Read the model definition and answer for the solid it produces. Units are mm, in the model's axes. A direction names the side the tool comes from. Give positions to 0.01 mm unless a question says otherwise; leave off trailing zeros. Write each loop counter-clockwise with the first axis right and the second up, starting at its lowest first coordinate (ties: lowest second). Pieces come first, ordered by that corner, then holes. Notation, with made-up numbers: (20.5, 34) - (65.5, 34) arc R6 cw to (65.5, 43) - close; hole circle Ø8 at (71, 61). An arc over 180 degrees is marked (long way). Use CSV: the item, a comma, the result in double quotes. Start each with the question number.
from build123d import *

# Parameters (mm, degrees)
SKETCH_1_R               = 4
EXTRUDE_1_DEPTH          = 2
SKETCH_6_R               = 6
EXTRUDE_3_DEPTH          = 1
SKETCH_2_R               = 0.5
CUT_EXTRUDE_1_DEPTH      = 2
PATTERN_CIRCULAR_1_COUNT = 3
CHAMFER_1_SIZE           = 0.5
EXTRUDE_START            = -2
EXTRUDE_4_DEPTH          = 2
HOLE_WIZARD_M3_1_D       = 3.4
SKETCH_11_R              = 3.5
CUT_EXTRUDE_3_DEPTH      = 1
CUT_EXTRUDE_4_DEPTH      = 29.574464124
FILLET_1_R               = 1
FILLET_2_R               = 1


with BuildPart() as part:
    # ｽｹｯﾁ1 → ﾎﾞｽ - 押し出し1 (new body)
    with BuildSketch(Plane.XY):
        with BuildLine():
            ThreePointArc((-4.5, -6), (7.5, 0), (-4.5, 6))
            ThreePointArc((-4.5, 6), (-7.5, 5), (-10.5, 6))
            ThreePointArc((-10.5, 6), (-22.5, 0), (-10.5, -6))
            ThreePointArc((-10.5, -6), (-7.5, -5), (-4.5, -6))
        make_face()
        Circle(SKETCH_1_R, mode=Mode.SUBTRACT)
    extrude(amount=EXTRUDE_1_DEPTH)

    # ｽｹｯﾁ6 → ﾎﾞｽ - 押し出し3 (add)
    with BuildSketch(Plane.XY.offset(2)):
        with Locations((-15, 0)):
            Circle(SKETCH_6_R)
    extrude(amount=EXTRUDE_3_DEPTH)

    # ｽｹｯﾁ2 → ｶｯﾄ - 押し出し1 (cut)
    with BuildSketch(Plane.XY.offset(3)):
        with Locations((-11.5, 0)):
            Circle(SKETCH_2_R)
    extrude(amount=-CUT_EXTRUDE_1_DEPTH, mode=Mode.SUBTRACT)

    # ｽｹｯﾁ4 → M3x0.5 ねじ穴1 (revolve, cut)
    with BuildSketch(Plane(origin=(-11.5, 0, 3), x_dir=(0, -1, 0), z_dir=(1, 0, 0))):
        Polygon((0, 0), (0, 3), (1.525, 3), (1.25, 2.725), (1.25, 0.025), (1.275, 0), align=None)
    m3x0_5_1 = revolve(axis=Axis((-11.5, 0, 9.35), (0, 0, -1)), mode=Mode.SUBTRACT)

    # 円形ﾊﾟﾀｰﾝ1: M3x0.5 ねじ穴1 ×3 about axis
    pattern_circular_1_axis = Axis((-15, 0, 0), (0, 0, 1))
    for i in range(1, PATTERN_CIRCULAR_1_COUNT):
        add(m3x0_5_1.rotate(pattern_circular_1_axis, i * 360 / PATTERN_CIRCULAR_1_COUNT), mode=Mode.SUBTRACT)

    # 面取り1
    chamfer_1_edges = [part.edges().sort_by_distance(p)[0] for p in [
        (-21, 0, 3),
    ]]
    chamfer(chamfer_1_edges, length=CHAMFER_1_SIZE)

    # ｽｹｯﾁ7 → ﾎﾞｽ - 押し出し4 (add)
    with BuildSketch(Plane.XY.offset(2).offset(EXTRUDE_START)):
        with BuildLine():
            ThreePointArc((-15.833333333, -7.453559925), (3.818813079, -17.078251277), (17.5, 0))
            ThreePointArc((17.5, 0), (3.818813079, 17.078251277), (-15.833333333, 7.453559925))
            ThreePointArc((-15.833333333, 7.453559925), (-13.027864045, 7.236067977), (-10.5, 6))
            ThreePointArc((-10.5, 6), (-7.5, 5), (-4.5, 6))
            ThreePointArc((-4.5, 6), (7.5, 0), (-4.5, -6))
            ThreePointArc((-4.5, -6), (-7.5, -5), (-10.5, -6))
            ThreePointArc((-10.5, -6), (-13.027864045, -7.236067977), (-15.833333333, -7.453559925))
        make_face()
    extrude(amount=EXTRUDE_4_DEPTH)

    # M3 すきま穴1 (through all)
    with Locations(Plane.XY.offset(2)):
        with Locations((-5, 8.660254038), (-5, -8.660254038), (10, 0)):
            Hole(HOLE_WIZARD_M3_1_D / 2)

    # ｽｹｯﾁ11 → ｶｯﾄ - 押し出し3 (cut)
    with BuildSketch(Plane.XY.offset(2)):
        with Locations((-5, 8.660254038)):
            Circle(SKETCH_11_R)
        with Locations((10, 0)):
            Circle(SKETCH_11_R)
        with Locations((-5, -8.660254038)):
            Circle(SKETCH_11_R)
    extrude(amount=-CUT_EXTRUDE_3_DEPTH, mode=Mode.SUBTRACT)

    # ｽｹｯﾁ12 → ｶｯﾄ - 押し出し4 (cut, through all)
    with BuildSketch(Plane.XY.offset(2)):
        with BuildLine():
            ThreePointArc((6.09375, 3.121091306), (7.83268098, 4.505854887), (10, 5))
            Line((10, 5), (12.539936204, 5))
            ThreePointArc((12.539936204, 5), (6.75, 11.691342951), (-1.939841083, 13.359903314))
            Line((-1.939841083, 13.359903314), (-0.669872981, 11.160254038))
            ThreePointArc((-0.669872981, 11.160254038), (-0.014155692, 9.036228152), (-0.343930642, 6.837887957))
            ThreePointArc((-0.343930642, 6.837887957), (-0.263339736, 5.947638581), (0.496931964, 5.477504781))
            ThreePointArc((0.496931964, 5.477504781), (2.75, 4.763139721), (4.495192308, 3.169108095))
            ThreePointArc((4.495192308, 3.169108095), (5.282475971, 2.745760389), (6.09375, 3.121091306))
        make_face()
        with BuildLine():
            ThreePointArc((-1.939841083, -13.359903314), (6.75, -11.691342951), (12.539936204, -5))
            Line((12.539936204, -5), (10, -5))
            ThreePointArc((10, -5), (7.83268098, -4.505854887), (6.09375, -3.121091306))
            ThreePointArc((6.09375, -3.121091306), (5.282475971, -2.745760389), (4.495192308, -3.169108095))
            ThreePointArc((4.495192308, -3.169108095), (2.75, -4.763139721), (0.496931964, -5.477504781))
            ThreePointArc((0.496931964, -5.477504781), (-0.263339736, -5.947638581), (-0.343930642, -6.837887957))
            ThreePointArc((-0.343930642, -6.837887957), (-0.014155692, -9.036228152), (-0.669872981, -11.160254038))
            Line((-0.669872981, -11.160254038), (-1.939841083, -13.359903314))
        make_face()
        with BuildLine():
            ThreePointArc((-5.749819358, 3.716796652), (-6.813042195, 4.000546107), (-7.788444419, 4.510003717))
            ThreePointArc((-7.788444419, 4.510003717), (-9, 0), (-7.788444419, -4.510003717))
            ThreePointArc((-7.788444419, -4.510003717), (-6.813042195, -4.000546107), (-5.749819358, -3.716796652))
            ThreePointArc((-5.749819358, -3.716796652), (-5.019136236, -3.201878191), (-4.992124271, -2.308396686))
            ThreePointArc((-4.992124271, -2.308396686), (-5.5, 0), (-4.992124271, 2.308396686))
            ThreePointArc((-4.992124271, 2.308396686), (-5.019136236, 3.201878191), (-5.749819358, 3.716796652))
        make_face()
    extrude(amount=-CUT_EXTRUDE_4_DEPTH, mode=Mode.SUBTRACT)

    # ﾌｨﾚｯﾄ1
    fillet_1_edges = [part.edges().sort_by_distance(p)[0] for p in [
        (-1.939841083, 13.359903314, 1),
        (12.539936204, 5, 1),
        (12.539936204, -5, 1),
        (-1.939841083, -13.359903314, 1),
        (-7.788444419, 4.510003717, 1),
        (-7.788444419, -4.510003717, 1),
    ]]
    fillet(fillet_1_edges, radius=FILLET_1_R)

    # ﾌｨﾚｯﾄ2
    fillet_2_edges = [part.edges().sort_by_distance(p)[0] for p in [
        (-15.833333333, 7.453559925, 1),
        (-15.833333333, -7.453559925, 1),
    ]]
    fillet(fillet_2_edges, radius=FILLET_2_R)


solid = part.part
(1) The part is cut by section A-A on x = 7.5. Write down the section's boundary in (y, z), plus the area to 3 significant figures.
(2) Consider probe 1 along X at (y, z) = (7.5, 1.25); probe 2 along X at (y, z) = (2, 0.1); probe 3 along Y at (x, z) = (-5, 0.55). Determine where each line is inside the solid, lowest interval first.
(3) Which of the six approach directions +Z, -Z, +X, -X, +Y, -Y give full straight-line access (tool end or side, diameter ignored) to faces 4 (the face through (12, 1, 1)), 5 (the face through (-1.15, -13, 0.99))?
(4) Given P1, Ø1.1, axis at x = 10.5, z = 0.5, coming from the +Y side; P2, Ø6.5, axis at x = -5, y = 8.66, coming from the +Z side; P3, Ø12, axis at x = 7.5, y = 5, coming from the +Z side, each flat-ended and moving along its own axis, determine where each tip first touches the part or whether it passes through.
(5) For a pull along Y with two mould halves and no side action, classify faces 1 (the face through (-9.46, -2.3, 2.25)), 2 (the face through (2, 4, 2)), 3 (the face through (-0.867, -3.905, 0.986)) as pulls with the +Y half, pulls with the -Y half, needs draft (parallel to the pull), parting line crosses it, or undercut.
(6) The part is cut by section D-D on z = 1.55. Give the number of separate pieces and of enclosed holes in the cut face, plus the area to 3 significant figures.
(7) The part is cut by section B-B on y = -14. Write down the section's boundary in (x, z).
Reported:
1,outline,"(-15.81, 0) - (-11.22, 0) - (-11.22, 2) - (-15.81, 2) - close; (-4.33, 0) - (4.33, 0) - (4.33, 2) - (2.45, 2) - (2.45, 1) - (-2.45, 1) - (-2.45, 2) - (-4.33, 2) - close; (11.22, 0) - (15.81, 0) - (15.81, 2) - (11.22, 2) - close"
1,area,"30.8 mm²"
2,probe 1,"-16 to -8.3, -1.7 to -0.14, 11.22 to 15.81"
2,probe 2,"-22.23 to -17.73, -15.77 to -8.77, -5.12 to -3.46, 3.46 to 17.39"
2,probe 3,"-16.77 to -10.36, -6.96 to -3.16, -2.29 to 2.29, 3.16 to 6.96, 10.36 to 16.77"
3,face 4,"+Z"
3,face 5,"+Z, -Z"
4,P1,"y = 14.4"
4,P2,"z = 1"
4,P3,"z = 2"
5,face 1,"parting line crosses it"
5,face 2,"needs draft"
5,face 3,"undercut"
6,separate pieces,"1"
6,enclosed holes,"10"
6,area,"640 mm²"
7,outline,"(-10.5, 0) - (10.5, 0) - (10.5, 2) - (-10.5, 2) - close"
